```python
from build123d import *

# Parameters (mm, degrees)
SKETCH1_W           = 130
SKETCH1_H           = 60
BOSS_EXTRUDE2_DEPTH = 50
SHELL1_T            = -2.5
CUT_EXTRUDE1_REACH  = 132
SKETCH2_R           = 8.75
SKETCH3_R           = 8.75
CUT_EXTRUDE2_DEPTH  = 61
SKETCH4_W           = 50
SKETCH4_H           = 7.5
CUT_EXTRUDE3_DEPTH  = 61
CUT_EXTRUDE4_DEPTH  = 61


with BuildPart() as part:
    # Sketch1 → Boss-Extrude2 (new body)
    with BuildSketch(Plane(origin=(0, 0, 0), x_dir=(1, 0, 0), z_dir=(0, 1, 0))):
        Rectangle(SKETCH1_W, SKETCH1_H)
    extrude(amount=BOSS_EXTRUDE2_DEPTH)

    # Shell1
    shell1_openings = [part.faces().sort_by_distance(p)[0] for p in [
        (0, 0, 0),
    ]]
    offset(amount=SHELL1_T, openings=shell1_openings, kind=Kind.INTERSECTION)

    # Sketch2 → Cut-Extrude1 (cut, up to next)
    with BuildSketch(Plane(origin=(65, 0, 0), x_dir=(0, 0, -1), z_dir=(1, 0, 0)), mode=Mode.PRIVATE) as cut_extrude1_sk1:
        with Locations((-13, 35)):
            Circle(SKETCH2_R)
    cut_extrude1_tool1 = extrude(cut_extrude1_sk1.sketch, amount=-CUT_EXTRUDE1_REACH, mode=Mode.PRIVATE) & part.part
    add(cut_extrude1_tool1.solids().sort_by_distance((65, 35, 13))[0], mode=Mode.SUBTRACT)
    # Sketch2 → Cut-Extrude1 (cut, up to next)
    with BuildSketch(Plane(origin=(65, 0, 0), x_dir=(0, 0, -1), z_dir=(1, 0, 0)), mode=Mode.PRIVATE) as cut_extrude1_sk2:
        with BuildLine():
            ThreePointArc((21.75, 35), (13, 43.75), (4.25, 35))
            ThreePointArc((4.25, 35), (13, 26.25), (21.75, 35))
        make_face()
    cut_extrude1_tool2 = extrude(cut_extrude1_sk2.sketch, amount=-CUT_EXTRUDE1_REACH, mode=Mode.PRIVATE) & part.part
    add(cut_extrude1_tool2.solids().sort_by_distance((65, 35, -13))[0], mode=Mode.SUBTRACT)

    # Sketch3 → Cut-Extrude2 (cut, through all)
    with BuildSketch(Plane.XY.offset(30)):
        with Locations((22.274243645, 35)):
            Circle(SKETCH3_R)
        with Locations((48.274243645, 35)):
            Circle(SKETCH3_R)
    extrude(amount=-CUT_EXTRUDE2_DEPTH, mode=Mode.SUBTRACT)

    # Sketch4 → Cut-Extrude3 (cut, through all)
    with BuildSketch(Plane(origin=(0, 0, -30), x_dir=(-1, 0, 0), z_dir=(0, 0, -1))):
        with Locations((27.140672083, 18.75)):
            Rectangle(SKETCH4_W, SKETCH4_H)
    extrude(amount=-CUT_EXTRUDE3_DEPTH, mode=Mode.SUBTRACT)

    # Sketch5 → Cut-Extrude4 (cut, through all)
    with BuildSketch(Plane(origin=(0, 0, -30), x_dir=(-1, 0, 0), z_dir=(0, 0, -1))):
        with BuildLine():
            Line((20.475756355, 50), (28.475756355, 50))
            ThreePointArc((28.475756355, 50), (24.475756355, 46), (20.475756355, 50))
        make_face()
    extrude(amount=-CUT_EXTRUDE4_DEPTH, mode=Mode.SUBTRACT)


solid = part.part
```
CAD build for the part. Positions are in the model's coordinates, mm. A direction names the side the tool comes from. Coordinates: 2 decimals unless noted, no trailing zeros. Order: outer loops, then holes, each group sorted by start corner. A loop starts at its lowest first (then second) coordinate and runs counter-clockwise, first axis right, second up. Notation, with made-up numbers: M 40.5,-16.75 L 99.5,-16.75 A21 ccw 99.5,-4.75 Z; hole C -11.75,-9.75 d4. An arc over 180 degrees is marked long. Write each question's results on one line, items separated by ' | '. Start each with the question number.
Q1. Drill centre lines: probe 1 along Z at (x, y) = (-39, 26); probe 2 along Y at (x, z) = (64, 13); probe 3 along X at (y, z) = (45.5, -0.5). Where is each one in solid material? Low to high. Write a range as from..to.
Q2. Cut at B-B (x = -45). List the corners of the cut face in (y, z), then the cut area to 3 significant figures.
Q3. Cut at A-A (y = 35). Count the separate pieces of the cut face and the enclosed holes in it, then the cut area to 4 significant figures.
Q4. Pull direction X, two halves, no side cores. Call faces 5 (the cylindrical face through (46.377, 26.458, -28.732)), 6 (the flat face through (-1, 25, 30)), 7 (the flat face through (65, 25, 0)): +X half, -X half, draft (parallel to the pull), parting line (faces both ways), or undercut.
Q5. Cut at C-C (z = 23.5). List the corners of the cut face in (x, y).
Q6. Flat gauge pins, fed straight in: P1, Ø14, axis at y = 35, z = 13, coming from the +X side; P2, Ø10.5, axis at x = 48.27, y = 35, coming from the -Z side. Where does each tip first touch, or does it go through?
Q7. Which spindle directions (+Z, -Z, +X, -X, +Y, -Y) get a long thin tool onto all of the face, cutting with end or side? Do faces 1 (the cylindrical face through (63.77, 26.46, 14.9)), 2 (the flat face through (-62.5, 23, 0)), 3 (the flat face through (-47, 50, 0)), 4 (the flat face through (-52.141, 19, -29)). Say none if no direction does.
Q8. Cut at D-D (z = -13). List the corners of the cut face in (x, y), then the cut area to 3 significant figures.
Found:
1) probe 1: -30..-27.5, 27.5..30 | probe 2: 0..26.25, 43.75..50 | probe 3: -65..-62.5, 62.5..65
2) outline: M 0,-30 L 15,-30 L 15,-27.5 L 0,-27.5 Z; M 0,27.5 L 15,27.5 L 15,30 L 0,30 Z; M 22.5,-30 L 50,-30 L 50,30 L 22.5,30 L 22.5,27.5 L 47.5,27.5 L 47.5,-27.5 L 22.5,-27.5 Z | area: 350 mm²
3) separate pieces: 6 | enclosed holes: 0 | area: 662.5 mm²
4) face 5: undercut | face 6: draft | face 7: +X half
5) outline: M -65,0 L -62.5,0 L -62.5,47.5 L -27.6,47.5 A4 cw -28.48,50 L -65,50 Z; M -21.35,47.5 L 62.5,47.5 L 62.5,0 L 65,0 L 65,50 L -20.48,50 A4 cw Z
6) P1: x = -62.5 | P2: through
7) face 1: +X | face 2: -Y | face 3: +Z, -Z, +X, -X, +Y | face 4: +Z, -Z
8) outline: M -65,0 L -62.5,0 L -62.5,47.5 L -27.6,47.5 A4 cw -28.48,50 L -65,50 Z; M -21.35,47.5 L 62.5,47.5 L 62.5,43.75 L 65,43.75 L 65,50 L -20.48,50 A4 cw Z; M 62.5,0 L 65,0 L 65,26.25 L 62.5,26.25 Z | area: 500 mm²
